Autodesk Inventor part; units mm, degrees
ref_plane "YZ Plane" through (0, 0, 0) normal (1, 0, 0) x (0, 1, 0)
ref_plane "XZ Plane" through (0, 0, 0) normal (0, 1, 0) x (-1, 0, 0)
ref_plane "XY Plane" through (0, 0, 0) normal (0, 0, 1) x (1, 0, 0)
sketch "Sketch1" plane through (0, 0, 0) normal (0, 1, 0) x (-1, 0, 0)
  circle A0 centre (0, 0) radius 105
  dimension "d0" = 210
extrude "Extrusion1" add sketch "Sketch1" along normal blind 10
sketch "Sketch2" plane through (0, 10, 0) normal (0, 1, 0) x (1, 0, 0)
  line L0 (-79.8594, -68.6516) -> (79.5179, -68.6516)
  line L1 (0, 0) -> (0, -80)
  line L2 (0, -80) -> (0, -60)
  line L3 (0, -60) -> (17.5, -60)
  line L4 (0, -60) -> (-17.5, -60)
  circle A0 centre (-17.5, -60) radius 2.5
  circle A1 centre (0, -60) radius 2.5
  circle A2 centre (17.5, -60) radius 2.5
  dimension "d4" = 80
  dimension "d5" = 20
  dimension "d6" = 17.5
  dimension "d7" = 17.5
  dimension "d8" = 5
  dimension "d9" = 5
  dimension "d10" = 5
extrude "Extrusion2" cut sketch "Sketch2" against normal blind 10
sketch "Sketch3" plane through (0, 10, 0) normal (0, 1, 0) x (1, 0, 0)
  circle A0 centre (0, 0) radius 2.5
  dimension "d13" = 5
extrude "Extrusion3" cut sketch "Sketch3" against normal blind 10
sketch "Sketch4" plane through (0, 10, 0) normal (0, 1, 0) x (1, 0, 0)
  circle A0 centre (0, 0) radius 2.5
  line L0 (0, 0) -> (0, 80)
  line L1 (-15, 80) -> (-15, 65)
  line L2 (-15, 65) -> (15, 65)
  line L3 (15, 65) -> (15, 95)
  line L4 (15, 95) -> (-15, 95)
  line L5 (-15, 95) -> (-15, 80)
  line L6 (0, 80) -> (-7.5, 80)
  line L7 (-7.5, 80) -> (7.5, 80)
  line L8 (7.5, 80) -> (7.5, 95)
  line L9 (7.5, 80) -> (7.5, 65)
  line L10 (-7.5, 80) -> (-7.5, 95)
  line L11 (-7.5, 80) -> (-7.5, 65)
  dimension "d20" = 15
  dimension "d21" = 15
  dimension "d22" = 30
  dimension "d23" = 30
  dimension "d24" = 7.5
  dimension "d25" = 15
extrude "Extrusion4" add sketch "Sketch4" along normal blind 30 contours L2 L11 L6 L0 | L0 L7 L9 L2 | L6 L10 L4 L8 L7
sketch "Sketch5" plane through (7.5, 10, -65) normal (1, 0, 0) x (0, 0, -1)
  line L0 (40, 0) -> (-170, 0)
  line L1 (40, 0) -> (15, 0)
  line L2 (15, 0) -> (15, 15)
  circle A0 centre (15, 15) radius 7.5
  line L3 (30, 0) -> (30, 30)
  arc A1 (30, 15) -> (0, 15) centre (15, 15) ccw
  line L4 (15, 15) -> (0, 15) construction
  line L5 (15, 15) -> (30, 15) construction
  line L6 (0, 0) -> (0, 30)
  line L7 (0, 15) -> (0, 30)
  line L8 (0, 30) -> (30, 30)
  line L9 (0, 30) -> (30, 30)
  line L10 (30, 30) -> (30, 15)
  point P0 (-65, -10)
  point P1 (15, 30)
  dimension "d28" = 25
  dimension "d29" = 15
  dimension "d30" = 15
  dimension "d31" = 180
extrude "Extrusion5" cut sketch "Sketch5" against normal blind 30 contours A1 L8 L3 | A1 L6 L8 | A0
sketch "Sketch6" plane through (7.5, 10, -65) normal (1, 0, 0) x (0, 0, -1)
  circle A0 centre (15, 15) radius 7.5
  circle A1 centre (15, 15) radius 5
  circle A2 centre (15, 15) radius 7.5
  point P0 (-65, -10)
  dimension "d34" = 10
extrude "Extrusion6" add sketch "Sketch6" against normal blind 15
sketch "Sketch7" plane through (7.5, 10, -65) normal (1, 0, 0) x (0, 0, -1)
  line L0 (0, 0) -> (30, 0)
  line L1 (0, 0) -> (30, 0)
  line L2 (30, 0) -> (30, 34.6991)
  line L3 (30, 34.6991) -> (0, 34.6991)
  line L4 (0, 34.6991) -> (0, 0)
  point P0 (-65, -10)
extrude "Extrusion7" cut sketch "Sketch7" against normal blind 15
sketch "Sketch8" plane through (0, 10, 0) normal (0, 1, 0) x (1, 0, 0)
  circle A0 centre (0, 0) radius 2.5
  line L0 (0, 0) -> (0, 100)
  line L1 (0, 100) -> (-10, 100)
  line L2 (-10, 100) -> (-20, 100)
  line L3 (-20, 100) -> (-20, 65)
  line L4 (-20, 65) -> (-10, 65)
  line L5 (-10, 65) -> (-10, 100)
  line L6 (0, 100) -> (10, 100)
  line L7 (10, 100) -> (20, 100)
  line L8 (20, 100) -> (20, 65)
  line L9 (20, 65) -> (10, 65)
  line L10 (10, 65) -> (10, 100)
  dimension "d42" = 100
  dimension "d43" = 10
  dimension "d44" = 10
  dimension "d45" = 35
  dimension "d46" = 10
  dimension "d47" = 10
  dimension "d48" = 35
extrude "Extrusion8" add sketch "Sketch8" along normal blind 35 contours L5 L4 L3 L2 | L7 L8 L9 L10
thicken "Thicken1" operation add thickness 5 both sides no extend neighbours yes toward (0, 1, 0) faces at (13.3333, 45, -88.3333)
thicken "Thicken2" operation add thickness 5 both sides no extend neighbours yes toward (0, 1, 0) faces at (-16.6667, 45, -88.3333)
sketch "Sketch10" plane through (20, 10, -65) normal (1, 0, 0) x (0, 0, -1)
  line L0 (0, 0) -> (35, 0)
  line L1 (0, 0) -> (17.5, 0)
  line L2 (17.5, 0) -> (17.5, 22.5)
  circle A0 centre (17.5, 22.5) radius 12.5
  circle A1 centre (17.5, 22.5) radius 17.5
  line L3 (35, 0) -> (35, 40)
  line L4 (0, 0) -> (0, 40)
  line L5 (0, 22.5) -> (0, 40)
  line L6 (35, 40) -> (0, 40)
  line L7 (0, 40) -> (35, 40)
  line L8 (35, 40) -> (35, 22.5)
  point P0 (-65, -10)
  point P1 (17.5, 40)
  dimension "d60" = 22.5
  dimension "d61" = 25
extrude "Extrusion9" cut sketch "Sketch10" against normal blind 40 contours L4 L6 A1 | L6 L3 A1 | A0
sketch "Sketch11" plane through (20, 10, -65) normal (1, 0, 0) x (0, 0, -1)
  line L0 (40, 0) -> (-170, 0)
  line L1 (35.2175, 0) -> (0.2175, 0)
  line L2 (0.2175, 0) -> (-34.7825, 0)
  line L3 (0.2175, 0) -> (40.2175, 0)
  circle A0 centre (40.2175, 17.5) radius 12.5
  circle A1 centre (40.2175, 17.5) radius 17.5
  line L4 (-34.7825, 0) -> (32.4725, 33.1928)
  point P0 (-65, -10)
  dimension "d73" = 35
  dimension "d74" = 35
  dimension "d75" = 40
  dimension "d78" = 35
sketch "Sketch12" plane through (-20, 10, -100) normal (-1, 0, 0) x (0, 0, 1)
  line L0 (205, 0) -> (-5, 0)
  line L1 (37.401, 0) -> (37.401, 45.2729)
  line L2 (37.401, 45.2729) -> (-3.1543, 48.8051)
  line L3 (-3.1543, 48.8051) -> (-3.1543, 0)
  line L4 (37.401, 0) -> (-3.1543, 0)
  point P0 (100, -10)
extrude "Extrusion10" cut sketch "Sketch12" against normal blind 40
extrude "Extrusion11" add sketch "Sketch11" against normal blind 40
sketch "Sketch13" plane through (0, 0, 0) normal (0, 0, 1) x (1, 0, 0)
  line L0 (105, 10) -> (-105, 10)
  line L1 (0, 10) -> (10, 10)
  line L2 (10, 10) -> (10, 48.8421)
  line L3 (20, 43.1928) -> (-20, 43.1928)
  line L4 (10, 48.8421) -> (-10, 48.8421)
  line L5 (-10, 48.8421) -> (-10, 10)
  line L6 (-10, 10) -> (10, 10)
  point P0 (0, 0)
  point P1 (-20, 10)
  point P2 (20, 10)
  dimension "d83" = 10
  dimension "d84" = 20
extrude "Extrusion12" cut sketch "Sketch13" against normal blind 150
sketch "Sketch14" plane through (20, 10, -65) normal (1, 0, 0) x (0, 0, -1)
  line L0 (38.0776, 0) -> (-34.7825, 0)
  line L1 (-34.7825, 0) -> (42.8397, 49.7383)
  line L2 (42.8397, 49.7383) -> (77.8644, 0)
  line L3 (77.8644, 0) -> (-34.7825, 0)
  point P0 (-65, -10)
extrude "Extrusion13" cut sketch "Sketch14" against normal blind 150
sketch "Sketch15" plane through (0, 10, 0) normal (0, 1, 0) x (1, 0, 0)
  circle A0 centre (0, 0) radius 2.5
  line L0 (0, 0) -> (0, 100)
  line L1 (0, 100) -> (-20, 100)
  line L2 (-20, 100) -> (-20, 65)
  line L3 (-20, 65) -> (-10, 65)
  line L4 (-10, 65) -> (-10, 100)
  line L5 (-10, 65) -> (10, 65)
  line L6 (10, 65) -> (20, 65)
  line L7 (20, 65) -> (20, 100)
  line L8 (20, 100) -> (10, 100)
  line L9 (10, 100) -> (10, 65)
  dimension "d89" = 100
  dimension "d90" = 20
  dimension "d91" = 35
  dimension "d92" = 10
  dimension "d93" = 20
  dimension "d94" = 10
  dimension "d95" = 35
  dimension "d96" = 10
extrude "Extrusion14" add sketch "Sketch15" along normal blind 40 contours L3 L2 L1 L4 | L9 L8 L7 L6
sketch "Sketch16" plane through (20, 10, -65) normal (1, 0, 0) x (0, 0, -1)
  line L0 (0, 40) -> (35, 40)
  line L1 (17.5, 40) -> (17.5, 22.5)
  circle A0 centre (17.5, 22.5) radius 12.5
  circle A1 centre (17.5, 22.5) radius 17.5
  line L2 (35, 0) -> (35, 40)
  line L3 (0, 0) -> (0, 40)
  line L4 (0, 22.5) -> (0, 40)
  line L5 (0, 40) -> (35, 40)
  line L6 (35, 40) -> (35, 22.5)
  point P0 (-65, -10)
  dimension "d99" = 17.5
  dimension "d100" = 25
extrude "Extrusion15" cut sketch "Sketch16" against normal blind 40 contours L0 A1 L3 | L0 L2 A1 | A0
sketch "Sketch18" plane through (0, 10, 0) normal (0, 1, 0) x (1, 0, 0)
  line L0 (-10, 65) -> (-20, 65)
  line L1 (10, 65) -> (10, 100)
  line L2 (-10, 65) -> (10, 65)
  line L3 (10, 65) -> (10, 111.2793)
  line L4 (10, 111.2793) -> (-10, 111.2793)
  line L5 (-10, 100) -> (-10, 65)
  line L6 (-10, 111.2793) -> (-10, 65)
  point P0 (0, 0)
extrude "Extrusion17" cut sketch "Sketch18" against normal blind 40
sketch "Sketch19" plane through (0, 10, 0) normal (0, 1, 0) x (1, 0, 0)
  circle A0 centre (0, 0) radius 2.5
  line L0 (0, 0) -> (0, -85)
  circle A1 centre (0, -85) radius 2.5
  circle A2 centre (17.5, -85) radius 2.5
  circle A3 centre (-17.5, -85) radius 2.5
  dimension "d119" = 85
  dimension "d120" = 5
  dimension "d121" = 5
  dimension "d122" = 5
extrude "Extrusion18" cut sketch "Sketch19" against normal blind 10 contours A1 | A2 | A3
sketch "Sketch20" plane through (0, 10, 0) normal (0, 1, 0) x (1, 0, 0)
  circle A0 centre (0, -60.0339) radius 2.5
  circle A1 centre (17.5, -60) radius 2.5
  circle A2 centre (17.5, -60) radius 2.5
  circle A3 centre (-17.5, -60) radius 2.5
  circle A4 centre (-17.5, -60) radius 2.5
  point P0 (0, 0)
  dimension "d125" = 5
  dimension "d126" = 5
  dimension "d127" = 5
extrude "Extrusion19" add sketch "Sketch20" against normal blind 10
sketch "Sketch21" plane through (0, 10, 0) normal (0, 1, 0) x (1, 0, 0)
  circle A0 centre (0, -62.5) radius 12.6485
  point P0 (0, 0)
extrude "Extrusion20" add sketch "Sketch21" against normal blind 10
sketch "Sketch28" plane through (0, 10, 0) normal (0, 1, 0) x (1, 0, 0)
  line L0 (0, 0) -> (0, 145)
  line L1 (0, 145) -> (-25, 145)
  line L2 (-25, 145) -> (-25, 58.6582)
  line L3 (-25, 58.6582) -> (25.7597, 58.6582)
  line L4 (25.7597, 58.6582) -> (25.7597, 145)
  line L5 (25.7597, 145) -> (0, 145)
  dimension "d165" = 145
  dimension "d166" = 25
extrude "Extrusion27" add sketch "Sketch28" against normal blind 10
sketch "Sketch29" plane through (0, 10, 0) normal (0, 1, 0) x (1, 0, 0)
  line L0 (0, 56.8176) -> (-28.7063, 61.8747)
  line L1 (-28.7063, 61.8747) -> (-21.0018, 105.6086)
  line L2 (-21.0018, 105.6086) -> (22.7568, 105.6086)
  line L3 (22.7568, 105.6086) -> (27.8138, 56.8176)
  line L4 (27.8138, 56.8176) -> (0, 56.8176)
  point P0 (0, 0)
extrude "Extrusion28" cut sketch "Sketch29" along normal blind 40
sketch "Sketch30" plane through (0, 10, 0) normal (0, 1, 0) x (1, 0, 0)
  line L0 (25.7597, 145) -> (-25, 145)
  line L1 (-25, 145) -> (-10, 145)
  line L2 (-10, 145) -> (10, 145)
  line L3 (0, 145) -> (-10, 145)
  line L4 (-10, 145) -> (-20, 145)
  line L5 (-20, 145) -> (-20, 110)
  line L6 (-20, 110) -> (-10, 110)
  line L7 (-10, 110) -> (-10, 145)
  line L8 (0, 145) -> (10, 145)
  line L9 (10, 145) -> (20, 145)
  line L10 (20, 145) -> (20, 110)
  line L11 (20, 110) -> (10, 110)
  line L12 (10, 110) -> (10, 145)
  point P0 (0, 0)
  dimension "d173" = 10
  dimension "d174" = 10
  dimension "d175" = 35
  dimension "d176" = 10
  dimension "d177" = 10
  dimension "d178" = 10
extrude "Extrusion29" add sketch "Sketch30" along normal blind 40
fillet "Fillet4" radius 17.5 4 edges at (15, 50, -145) (15, 50, -110) (-15, 50, -110) (-15, 50, -145)
sketch "Sketch31" plane through (0, 10, 0) normal (0, 1, 0) x (1, 0, 0)
  line L0 (-25, 145) -> (25.7597, 145)
  line L1 (0, 145) -> (-25, 145)
  line L2 (0, 145) -> (25, 145)
  circle A0 centre (0, 0) radius 2.5
  circle A1 centre (0, 0) radius 105
  line L3 (25, 145) -> (25, 101.9804)
  line L4 (25, 145) -> (25.7597, 145)
  line L5 (25.7597, 145) -> (25.7597, 101.7911)
  dimension "d182" = 25
  dimension "d183" = 25
  dimension "d184" = 210
extrude "Extrusion30" cut sketch "Sketch31" against normal blind 40 contours L0 L5 A1 L3
sketch "Sketch32" plane through (20, 10, -110) normal (1, 0, 0) x (0, 0, -1)
  arc A0 (35, 22.5) -> (0, 22.5) centre (17.5, 22.5) ccw
  circle A1 centre (17.5, 22.5) radius 12.5
  point P0 (-110, -10)
  dimension "d187" = 25
extrude "Extrusion31" cut sketch "Sketch32" against normal blind 40
fillet "Fillet5" radius 5 4 edges at (25, 5, -145) (25, 5, -101.9804) (-25, 5, -145) (-25, 5, -101.9804)
sketch "Sketch33" plane through (0, 10, 0) normal (0, 1, 0) x (1, 0, 0)
  line L0 (10, 110) -> (20, 110)
  line L1 (10, 110) -> (-10, 110)
  line L2 (-10, 110) -> (-10, 145)
  line L3 (-10, 145) -> (10, 145)
  line L4 (10, 110) -> (10, 145)
  line L5 (10, 145) -> (10, 110)
  point P0 (0, 0)
  dimension "d191" = 20
  dimension "d192" = 35
extrude "Extrusion32" cut sketch "Sketch33" against normal blind 40
properties part number "Base do telescópio"
For this review, take the finished solid that the model builds, in its own axes (mm). A direction names the side the tool comes from. Round coordinates to 2 decimals unless told otherwise and drop trailing zeros. Write each loop counter-clockwise with the first axis right and the second up, starting at its lowest first coordinate (ties: lowest second). Pieces come first, ordered by that corner, then holes. Notation, with made-up numbers: (61.5, -31.5) -> (82.5, -31.5) arc R6 ccw to (82.5, -26.5) -> close; hole circle Ø8 at (17, 54). An arc over 180 degrees is marked (long way). Use one line per item in the form item = value.
1) Tool access review of faces 1 (the flat face through (10, 19.8, -127.3)), 2 (the flat face through (25, 5, -123)), 3 (the flat face through (-20, 21, -120)): name each direction out of +Z, -Z, +X, -X, +Y, -Y from which nothing blocks a thin tool from reaching the whole face with its end or side.
Found:
face_1 = -Z, +Y, -Y
face_2 = -Z, +X, +Y, -Y
face_3 = +Z, -Z, -X, +Y
2) Take a section at C-C, the plane x = -67. Write out the cut boundary in (y, z), and give its area (3 significant figures).
Found:
outline = (0, -80.85) -> (10, -80.85) -> (10, 80.85) -> (0, 80.85) -> close
area = 1,620 mm2
3) Take a section at A-A, the plane y = 25. Write out the cut boundary in (x, z), and give its area (3 significant figures).
Found:
outline = (-20, -145) -> (-10, -145) -> (-10, -137.5) -> (-20, -137.5) -> close; (-20, -117.5) -> (-10, -117.5) -> (-10, -110) -> (-20, -110) -> close; (10, -145) -> (20, -145) -> (20, -137.5) -> (10, -137.5) -> close; (10, -117.5) -> (20, -117.5) -> (20, -110) -> (10, -110) -> close
area = 300 mm2
4) Take a section at B-B, the plane z = -10.5. Write out the cut boundary in (x, y), and give its area (3 significant figures).
Found:
outline = (-104.47, 0) -> (104.47, 0) -> (104.47, 10) -> (-104.47, 10) -> close
area = 2,090 mm2
5) To check wall thickness, follow L1, parallel to Y at x = -12, z = -127; L2, parallel to X at y = 8, z = 0; L3, parallel to Z at x = 0, y = 6.25. State the ranges of each line that lie inside material, in increasing order. Write a range as from..to.
Found:
L1 = 0..20.01, 44.99..49.99
L2 = -105..-2.5, 2.5..105
L3 = -110..-2.5, 2.5..82.5, 87.5..105
6) Clearance check with flat-ended pins moving along their axes: pin 1 (17.5 mm diameter, centred on y = 31, z = -130, fed in from +X); pin 2 (6 mm diameter, centred on x = 0, z = 85, fed in from +Y); pin 3 (8 mm diameter, centred on x = 3, y = 4.5, fed in from -Z); pin 4 (4 mm diameter, centred on y = 17, z = -117.5, fed in from +X). State where each tip first meets the part, or that it passes through.
Found:
pin_1 = through
pin_2 = 10
pin_3 = -110
pin_4 = 20
7) Mouldability with a two-part tool opening along Y and no side actions: class faces 4 (the flat face through (15, 16, -145)), 5 (the cylindrical face through (-15.07, 45.01, -139.74)), 6 (the cylindrical face through (15.07, 36.255, -139.423)) as +Y half, -Y half, draft (parallel to the pull), parting line (faces both ways), or undercut.
Found:
face_4 = draft
face_5 = +Y half
face_6 = undercut
